from build123d import *

# Parameters (mm, degrees)
ESQUISSE1_R        = 1.5
BOSS_EXTRU_1_DEPTH = 1


with BuildPart() as part:
    # Esquisse1 → Boss.-Extru.1 (new body)
    with BuildSketch(Plane.XY):
        with BuildLine():
            Line((0, 0), (20, 0))
            Line((20, 0), (20, 10))
            Line((20, 10), (11.392388155, 10))
            ThreePointArc((11.392388155, 10), (10.006568857, 10.925974851), (10.331727984, 12.560660172))
            Line((10.331727984, 12.560660172), (17.335533906, 19.564466094))
            ThreePointArc((17.335533906, 19.564466094), (17.335533906, 26.635533906), (10.264466094, 26.635533906))
            Line((10.264466094, 26.635533906), (0, 16.371067812))
            Line((0, 16.371067812), (0, 0))
        make_face()
        with Locations((5, 5)):
            Circle(ESQUISSE1_R, mode=Mode.SUBTRACT)
        with Locations((15, 5)):
            Circle(ESQUISSE1_R, mode=Mode.SUBTRACT)
        with Locations((6, 15.3)):
            Circle(ESQUISSE1_R, mode=Mode.SUBTRACT)
        with Locations((13.071067812, 22.371067812)):
            Circle(ESQUISSE1_R, mode=Mode.SUBTRACT)
    extrude(amount=BOSS_EXTRU_1_DEPTH)


solid = part.part
The listing builds one solid part. Answer for the finished solid, in the listing's coordinates (mm). A direction names the side the tool comes from. Coordinates: 2 decimals unless noted, no trailing zeros. Write each loop counter-clockwise with the first axis right and the second up, starting at its lowest first coordinate (ties: lowest second). Pieces come first, ordered by that corner, then holes. Notation, with made-up numbers: M -12,8 L 16,8 A16 cw 16,32 Z; hole C 16,34.25 d2. An arc over 180 degrees is marked long. Put each result on its own line as item: value. Start each with the question number.
1. A cutting plane is placed at A-A on y = 5. Write down the section's boundary in (x, z).
2. Consider line 1 (X direction, y = 4.75, z = 0.3); line 2 (Y direction, x = 15, z = 0.65); line 3 (Y direction, x = 5, z = 0.25). Determine where each line is inside the solid, lowest interval first. Write a range as from..to.
3. A cutting plane is placed at D-D on x = 13.8. Write down the section's boundary in (y, z).
4. For a pull along Y with two mould halves and no side action, classify faces 3 (the flat face through (5.204, 21.575, 0.493)), 4 (the cylindrical face through (17.41, 26.56, 0.49)), 5 (the flat face through (10, 14, 1)) as pulls with the +Y half, pulls with the -Y half, needs draft (parallel to the pull), parting line crosses it, or undercut.
5. A cutting plane is placed at C-C on z = 0.4. Write down the section's boundary in (x, y), then the cut area to 3 significant figures.
6. Which of the six approach directions +Z, -Z, +X, -X, +Y, -Y give full straight-line access (tool end or side, diameter ignored) to faces 1 (the flat face through (0, 8.3, 0.5)), 2 (the flat face through (15.8, 10, 0.5))?
7. A cutting plane is placed at B-B on y = 23.1. Write down the section's boundary in (x, z).
Resolved:
1. outline: M 0,0 L 3.5,0 L 3.5,1 L 0,1 Z; M 6.5,0 L 13.5,0 L 13.5,1 L 6.5,1 Z; M 16.5,0 L 20,0 L 20,1 L 16.5,1 Z
2. line 1: x = 0..3.52, 6.48..13.52, 16.48..20
2. line 2: y = 0..3.5, 6.5..10, 17.23..27.95
2. line 3: y = 0..3.5, 6.5..14.18, 16.42..21.37
3. outline: M 0,0 L 4.1,0 L 4.1,1 L 0,1 Z; M 5.9,0 L 10,0 L 10,1 L 5.9,1 Z; M 16.03,0 L 21.06,0 L 21.06,1 L 16.03,1 Z; M 23.68,0 L 28.1,0 L 28.1,1 L 23.68,1 Z
4. face 3: pulls with the +Y half
4. face 4: undercut
4. face 5: needs draft
5. outline: M 0,0 L 20,0 L 20,10 L 11.39,10 A1.5 cw 10.33,12.56 L 17.34,19.56 A5 ccw 10.26,26.64 L 0,16.37 Z; hole C 5,5 d3; hole C 6,15.3 d3; hole C 13.07,22.37 d3; hole C 15,5 d3
5. area: 379 mm2
6. face 1: +Z, -Z, -X, +Y, -Y
6. face 2: +Z, -Z, +X
7. outline: M 6.73,0 L 11.76,0 L 11.76,1 L 6.73,1 Z; M 14.38,0 L 18.8,0 L 18.8,1 L 14.38,1 Z
